Input: dimensioned drawing with shaded views. Units: mm. Origin: part minimum x, y, z. Coordinates: 2 decimals unless noted, no trailing zeros. Order: outer loops, then holes, each group sorted by start corner. A loop starts at its lowest first (then second) coordinate and runs counter-clockwise, first axis right, second up.
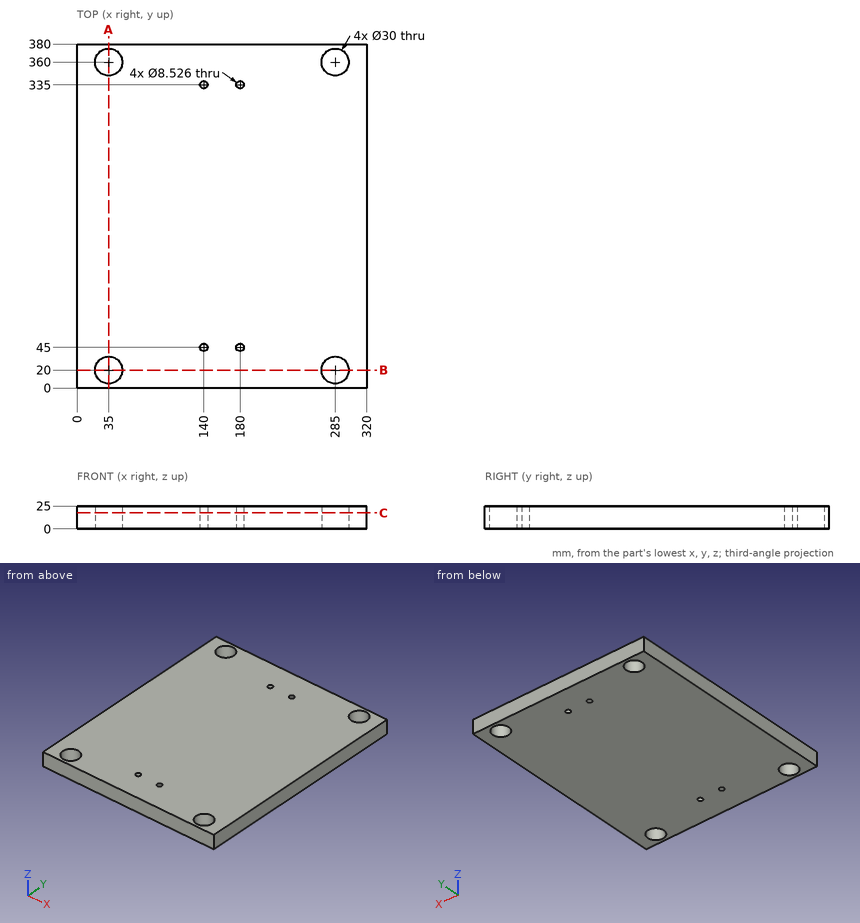
1. Section query B-B on y = 20. Return loops of the section in (x, z), plus the area to 3 significant figures.
Findings:
outline: (0, 0) - (20, 0) - (20, 25) - (0, 25) - close; (50, 0) - (270, 0) - (270, 25) - (50, 25) - close; (300, 0) - (320, 0) - (320, 25) - (300, 25) - close
area: 6,500 mm2
2. Section query C-C on z = 17.5. Count the separate pieces of the cut face and the enclosed holes in it, plus the area to 3 significant figures.
Findings:
separate pieces: 1
enclosed holes: 8
area: 119,000 mm2
3. Section query A-A on x = 35. Return loops of the section in (y, z), plus the area to 3 significant figures.
Findings:
outline: (0, 0) - (5, 0) - (5, 25) - (0, 25) - close; (35, 0) - (345, 0) - (345, 25) - (35, 25) - close; (375, 0) - (380, 0) - (380, 25) - (375, 25) - close
area: 8,000 mm2
4. Ray query, line 1 (X direction, y = 20, z = 19); line 2 (Y direction, x = 285, z = 19); line 3 (Y direction, x = 140, z = 6.5). Return the intervals inside material, ascending.
Findings:
line 1: x = 0 to 20, 50 to 270, 300 to 320
line 2: y = 0 to 5, 35 to 345, 375 to 380
line 3: y = 0 to 40.74, 49.26 to 330.74, 339.26 to 380
5. Pin query (flat end, axial travel): P1, Ø24, axis at x = 35, y = 360, coming from the -Z side. Return the tip coordinate at first contact, or that it passes through.
Findings:
P1: passes through
